Model file for the job. Use its own axes, mm. A direction names the side the tool comes from. Coordinates: 2 decimals unless noted, no trailing zeros. Write each loop counter-clockwise with the first axis right and the second up, starting at its lowest first coordinate (ties: lowest second). Pieces come first, ordered by that corner, then holes. Notation, with made-up numbers: M 28.25,38 L 34.25,38 A27 ccw 34.25,54 Z; hole C -37.5,27.5 d7. An arc over 180 degrees is marked long. Put each result on its own line as item: value. Start each with the question number.
Q1. Cut at B-B (x = 0). Write the cut outline in (y, z).
Q2. Drill centre lines: line 1 along Z through (x, y) = (-15, 0); line 2 along Z through (x, y) = (0, -13); line 3 along X through (y, z) = (33, 20). Where is each one in solid material? Low to high.
Q3. Pull direction Z, two halves, no side cores. Call faces 1 (the flat face through (-1, 1, 100)), 2 (the cylindrical face through (-8.671, 0.314, 11.066)), 3 (the cylindrical face through (100.31, -5.8, 95.33)), 4 (the flat face through (-23, 50, 16)): pulls with the +Z half, pulls with the -Z half, needs draft (parallel to the pull), parting line crosses it, or undercut.
Q4. Cut at A-A (y = 0). Write the cut outline in (x, z), then the cut area to 3 significant figures.
Q5. Which spindle directions (+Z, -Z, +X, -X, +Y, -Y) get a long thin tool onto all of the face, cutting with end or side? Do faces 5 (the flat face through (50, -29, 14)), 6 (the flat face through (150, -30, 78)). Say none if no direction does.
Q6. Drop flat-ended pins along their axis: pin 1 (10 mm diameter, centred on x = 110, z = 77.5, fed in from -Y); pin 2 (10 mm diameter, centred on x = 63.5, y = -17, fed in from +Z); pin 3 (1.5 mm diameter, centred on x = 129.5, y = -6.5, fed in from +Z). Give the stop position or say it passes through.
```python
from build123d import *

# Parameters (mm, degrees)
F0_W     = 100
F0_H     = 100
F1_DEPTH = 100
F2_R     = 40
F3_DEPTH = 100.001
F4_R     = 40
F5_DEPTH = 100.001
F2_R_2   = 44.5208759626
F6_DEPTH = 100
F7_R     = 2


with BuildPart() as f1:
    # F0 (on Top) → F1 (new body)
    with BuildSketch(Plane.XY):
        Rectangle(F0_W, F0_H)
    extrude(amount=F1_DEPTH)

    # F2 (on face) → F3 (cut, through all)
    with BuildSketch(Plane.YZ.offset(50)):
        with Locations((0, 51.1895758084)):
            Circle(F2_R)
    extrude(amount=-F3_DEPTH, mode=Mode.SUBTRACT)

    # F4 (on face) → F5 (cut, through all)
    with BuildSketch(Plane.XZ.offset(50)):
        with Locations((0, 50.114749205)):
            Circle(F4_R)
    extrude(amount=-F5_DEPTH, mode=Mode.SUBTRACT)

    # F2 (on face) → F6 (join)
    with BuildSketch(Plane.YZ.offset(50)):
        with Locations((0, 51.1895758084)):
            Circle(F2_R_2)
        with Locations((0, 51.1895758084)):
            Circle(F2_R, mode=Mode.SUBTRACT)
    extrude(amount=F6_DEPTH)

    # F7
    f7_edges = [f1.edges().sort_by_distance(p)[0] for p in [
        (0, -50, 100),
        (50, 0, 100),
        (0, 50, 100),
        (-50, 0, 100),
        (50, -50, 50),
        (50, 0, 0),
        (50, 50, 50),
        (50, -44.520876, 51.189576),
        (-50, -50, 50),
        (0, -50, 0),
        (-40, -50, 50.114749),
    ]]
    fillet(f7_edges, radius=F7_R)


solid = f1.part
```
Computed values:
1. outline: M -50,2 A2 ccw -48,0 L 50,0 L 50,10.11 L -48,10.11 A2 ccw -50,8.11 Z; M -50,92.11 A2 ccw -48,90.11 L -9.21,90.11 A40 cw 9.21,90.11 L 50,90.11 L 50,98 A2 ccw 48,100 L -48,100 A2 ccw -50,98 Z
2. line 1: 0 to 11.19, 91.19 to 100
2. line 2: 0 to 10.11, 90.11 to 100
2. line 3: -50 to -26.33, 26.33 to 50.34
3. face 1: pulls with the +Z half
3. face 2: undercut
3. face 3: parting line crosses it
3. face 4: needs draft
4. outline: M -50,0 L 48,0 A2 ccw 50,2 L 50,4.67 A2 cw 52,6.67 L 150,6.67 L 150,11.19 L 9.21,11.19 A40 cw -9.21,11.19 L -50,11.19 Z; M -50,91.19 L 150,91.19 L 150,95.71 L 52,95.71 A2 cw 50,97.71 L 50,98 A2 ccw 48,100 L -48,100 A2 ccw -50,98 Z
4. area: 2,890 mm2
5. face 5: +X
5. face 6: +Z, -Z, +X, +Y, -Y
6. pin 1: y = -39.09
6. pin 2: z = 94.06
6. pin 3: z = 95.34
